Could you check a few things on this drawing? It's one solid part, dimensions in mm from its lowest x, y, z. A direction names the side the tool comes from. Round coordinates to 2 decimals unless told otherwise and drop trailing zeros. Loops run counter-clockwise (first coordinate to the right, second up) from the corner with the lowest first, then second, coordinate; pieces in that order, holes last.
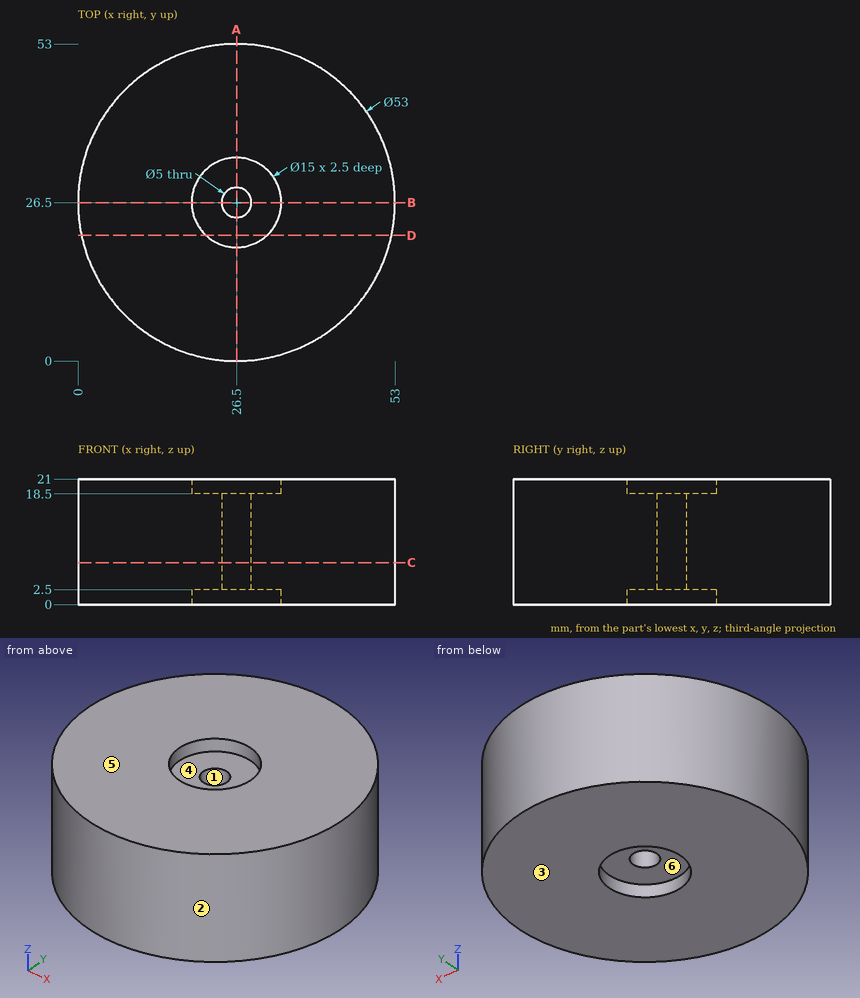
(1) We'd pull the mould along Y, two halves only. Please class the marked faces 1, 2 and 3: released by +Y, released by -Y, zero draft, split by the parting line, or undercut.
(2) For pin 1 (2 mm diameter, centred on y = 33.5, z = 10, fed in from -X); pin 2 (1 mm diameter, centred on y = 11, z = 12.5, fed in from +X); pin 3 (3 mm diameter, centred on x = 34.5, z = 9, fed in from -Y), each with a flat end and sliding along its axis, tell me the tip position at first contact or that it passes through.
(3) Which directions (+Z, -Z, +X, -X, +Y, -Y) give clear straight access to the entire face, cutting with the end or side of a thin tool? Please do the marked faces 4, 5 and 6.
(4) Suppose I cut it at C-C (z = 7). Write out the boundary of the cut face in (x, y).
(5) Suppose I cut it at A-A (x = 26.5). Write out the boundary of the cut face in (y, z).
(6) Suppose I cut it at D-D (y = 21). Write out the boundary of the cut face in (x, z), then the cut area to 3 significant figures.
(7) If I drill on line 1 (Y direction, x = 26.5, z = 19.25); line 2 (Z direction, x = 24.5, y = 29); line 3 (Y direction, x = 24.5, z = 12), over which ranges is the centre line in solid material (lowest first)?
Check result:
1. face 1: undercut
1. face 2: split by the parting line
1. face 3: zero draft
2. pin 1: stops at x = 0.69
2. pin 2: stops at x = 48.35
2. pin 3: stops at y = 0.81
3. face 4: +Z
3. face 5: +Z, +X, -X, +Y, -Y
3. face 6: -Z
4. outline: circle Ø53 at (26.5, 26.5); hole circle Ø5 at (26.5, 26.5)
5. outline: (0, 0) - (19, 0) - (19, 2.5) - (24, 2.5) - (24, 18.5) - (19, 18.5) - (19, 21) - (0, 21) - close; (29, 2.5) - (34, 2.5) - (34, 0) - (53, 0) - (53, 21) - (34, 21) - (34, 18.5) - (29, 18.5) - close
6. outline: (0.58, 0) - (21.4, 0) - (21.4, 2.5) - (31.6, 2.5) - (31.6, 0) - (52.42, 0) - (52.42, 21) - (31.6, 21) - (31.6, 18.5) - (21.4, 18.5) - (21.4, 21) - (0.58, 21) - close
6. area: 1,040 mm2
7. line 1: y = 0 to 19, 34 to 53
7. line 2: z = 2.5 to 18.5
7. line 3: y = 0.08 to 25, 28 to 52.92
